The model under review builds one solid part; all positions refer to its coordinate system, in mm. A direction names the side the tool comes from. Round coordinates to 2 decimals unless told otherwise and drop trailing zeros. Order: outer loops, then holes, each group sorted by start corner. A loop starts at its lowest first (then second) coordinate and runs counter-clockwise, first axis right, second up.
1) Consider section A-A (z = 46.5). Give the boundary of the cut face in (x, y) (3 decimals).
2) Clearance check with flat-ended pins moving along their axes: P1, Ø1.5, axis at x = -3.5, y = -4, coming from the +Z side; P2, Ø7.5, axis at x = 0, y = 0, coming from the -Z side; P3, Ø6, axis at x = 3.5, z = 40, coming from the +Y side; P4, Ø1.5, axis at y = 1, z = 30, coming from the -X side. State where each tip first meets the part, or that it passes through.
3) Machinability: for faces 1 (the face through (-0.69, 3.1, 28.55)), 2 (the face through (0.18, 0.79, 70.55)), which of the approach directions +Z, -Z, +X, -X, +Y, -Y give a long, thin tool a straight path to every point of the face, cutting with its end or side? Answer none if there is none.
4) To check wall thickness, follow L1, parallel to X at y = 0, z = 17.5 (3 decimals); L2, parallel to Y at x = 5.5, z = 14. State the ranges of each line that lie inside material, in increasing order.
5) Consider section B-B (z = 66.5). Give the boundary of the cut face in (x, y).
from build123d import *

# Parameters (mm, degrees)
F0_R     = 6.35
F1_DEPTH = 64.77
F5_R     = 3.175
F6_DEPTH = 57.912
F7_R     = 5.08


with BuildPart() as f1:
    # F0 (on Top) → F1 (new body)
    with BuildSketch(Plane.XY):
        Circle(F0_R)
    extrude(amount=F1_DEPTH)

    # F3 (on Front) → F4 (revolve)
    with BuildSketch(Plane.XZ):
        Polygon((0, 64.77), (0, 69.791943), (-2.845018, 72.444359), (-5.728471, 70.633823), (-6.35, 64.77), align=None)
    revolve(axis=Axis((0, 0, 36.195), (0, 0, 1)))

    # F5 (on face) → F6 (cut)
    with BuildSketch(Plane(origin=(0, 0, 0), x_dir=(1, 0, 0), z_dir=(0, 0, -1))):
        Circle(F5_R)
    extrude(amount=-F6_DEPTH, mode=Mode.SUBTRACT)

    # F7
    f7_edges = [f1.edges().sort_by_distance(p)[0] for p in [
        (5.728471, 0, 70.633823),
    ]]
    fillet(f7_edges, radius=F7_R)


solid = f1.part
Answer below:
1. outline: circle Ø12.7 at (0, 0); hole circle Ø6.35 at (0, 0)
2. P1: stops at z = 71.2
2. P2: stops at z = 0
2. P3: stops at y = 6.33
2. P4: stops at x = -6.35
3. face 1: -Z
3. face 2: +Z
4. L1: x = -6.35 to -3.175, 3.175 to 6.35
4. L2: y = -3.17 to 3.17
5. outline: circle Ø12.33 at (0, 0)
